Check sheet for the modelled part. Datum: model origin and axes. Units: mm. A direction names the side the tool comes from. Give positions to 0.01 mm unless a question says otherwise; leave off trailing zeros. Write each loop counter-clockwise with the first axis right and the second up, starting at its lowest first coordinate (ties: lowest second). Pieces come first, ordered by that corner, then holes. Notation, with made-up numbers: (-33, 66.25) -> (-8, 66.25) arc R19 cw to (-8, 99.25) -> close; hole circle Ø9 at (-10, -38.5). An arc over 180 degrees is marked (long way). Use a Markdown table: item, result. Add a question column.
1. Release check for a two-part mould opening along X. For faces 1 (the flat face through (2, 12, 15.875)), 2 (the cylindrical face through (21.199, 6.676, 7.826)), 3 (the cylindrical face through (-0.166, 20.637, 7.826)) record: released by +X, released by -X, zero draft, split by the parting line, or undercut.
2. Scan lines: probe 1 along Y at (x, z) = (-0.5, 5.25); probe 2 along X at (y, z) = (8.5, 3.5); probe 3 along X at (y, z) = (3, 14.25). Record each from-to range of solid material in increasing order. Write a range as [from, to].
3. Cross-section at D-D (y = 3). Enter the section's corners in (x, z) (3 decimals).
4. Cross-section at A-A (y = 10.5). Count the separate pieces of the cut face and the enclosed holes in it, then the cut area to 3 significant figures.
5. Cross-section at B-B (x = -5). Enter the section's corners in (y, z) (3 decimals).
6. Gauge pin test, flat ends, axial feed: P1, Ø2, axis at y = 1.5, z = 13.5, coming from the -X side; P2, Ø4, axis at y = -10.5, z = 11.5, coming from the -X side; P3, Ø3, axis at y = -17, z = 8, coming from the +X side. Record the tip position at first contact, or that the pin passes through.
7. Set-up check for faces 4 (the cylindrical face through (10.078, 10.477, 14.265)), 5 (the flat face through (-10, 10, 3.175)), 6 (the cylindrical face through (15.45, 13.31, 6.26)): record each of +Z, -Z, +X, -X, +Y, -Y from which the full face is reachable in a straight line by a thin tool's end or side.
from build123d import *

# Parameters (mm, degrees)
F0_R            = 22.225
F0_R_2          = 2.15265
F1_DEPTH        = 15.875
F4_R            = 3.96875
F5_DEPTH        = 12.7
F6_R            = 3.96875
F7_DEPTH        = 12.7
F9_DEPTH        = 15.875
F9_COPIES_COUNT = 4


# Not quite as in the source:
# - a pattern or mirror of a feature is missing from the dataset's text; its kind, count and spacing are read off the source's solid


with BuildPart() as f1:
    # F0 (on Top) → F1 (new body)
    with BuildSketch(Plane.XY):
        Circle(F0_R)
        with Locations((-11.7865861589, -11.7865861589)):
            Circle(F0_R_2, mode=Mode.SUBTRACT)
        with Locations((11.7865861589, -11.7865861589)):
            Circle(F0_R_2, mode=Mode.SUBTRACT)
        with Locations((-11.7865861589, 11.7865861589)):
            Circle(F0_R_2, mode=Mode.SUBTRACT)
        with BuildLine():
            ThreePointArc((0, 11.1125), (7.8577241059, 7.8577241059), (11.1125, 0))
            ThreePointArc((11.1125, 0), (-7.8577241059, -7.8577241059), (0, 11.1125))
        make_face(mode=Mode.SUBTRACT)
        with Locations((11.7865861589, 11.7865861589)):
            Circle(F0_R_2, mode=Mode.SUBTRACT)
    extrude(amount=F1_DEPTH)

    # F4 (on face) → F5 (cut, through all)
    with BuildSketch(Plane(origin=(0, 0, 0), x_dir=(1, 0, 0), z_dir=(0, 0, -1))):
        with Locations((11.7865861589, -11.7865861589)):
            Circle(F4_R)
        with Locations((-11.7865861589, 11.7865861589)):
            Circle(F4_R)
    extrude(amount=-F5_DEPTH, mode=Mode.SUBTRACT)

    # F6 (on face) → F7 (cut, through all)
    with BuildSketch(Plane.XY.offset(15.875)):
        with Locations((-11.7865861589, 11.7865861589)):
            Circle(F6_R)
        with Locations((11.7865861589, -11.7865861589)):
            Circle(F6_R)
    extrude(amount=-F7_DEPTH, mode=Mode.SUBTRACT)

    # F8 (on face) → F9 (cut, through all)
    with BuildSketch(Plane(origin=(0, 0, 0), x_dir=(1, 0, 0), z_dir=(0, 0, -1))):
        with BuildLine():
            ThreePointArc((-11.229543123, 17.3148424047), (-8.0281867, 15.8788163052), (-6.3255746232, 12.8109235396))
            ThreePointArc((-6.3255746232, 12.8109235396), (0, 14.2875), (6.3255746232, 12.8109235396))
            ThreePointArc((6.3255746232, 12.8109235396), (8.0281867, 15.8788163052), (11.229543123, 17.3148424047))
            ThreePointArc((11.229543123, 17.3148424047), (0, 20.6375), (-11.229543123, 17.3148424047))
        make_face()
    f9 = extrude(amount=-F9_DEPTH, mode=Mode.SUBTRACT)

    # F9_copies: F9 ×4 about axis
    f9_copies_axis = Axis((0, 0, 0), (0, 0, 1))
    for i in range(1, F9_COPIES_COUNT):
        add(f9.rotate(f9_copies_axis, i * 360 / F9_COPIES_COUNT), mode=Mode.SUBTRACT)


solid = f1.part
Worked answers:
| question | item | result |
|---|---|---|
| 1 | face 1 | zero draft |
| 1 | face 2 | split by the parting line |
| 1 | face 3 | undercut |
| 2 | probe 1 | y = [-22.22, -20.63], [-14.28, -11.1], [11.1, 14.28], [20.63, 22.22] |
| 2 | probe 2 | x = [-20.54, -18.81], [-16.27, -14.01], [-9.56, -7.16], [7.16, 9.56], [14.01, 16.27], [18.81, 20.54] |
| 2 | probe 3 | x = [-22.02, -20.42], [-13.97, -10.7], [10.7, 13.97], [20.42, 22.02] |
| 3 | outline | (-22.022, 0) -> (-20.418, 0) -> (-20.418, 15.875) -> (-22.022, 15.875) -> close; (-13.969, 0) -> (-10.7, 0) -> (-10.7, 15.875) -> (-13.969, 15.875) -> close; (10.7, 0) -> (13.969, 0) -> (13.969, 15.875) -> (10.7, 15.875) -> close; (20.418, 0) -> (22.022, 0) -> (22.022, 15.875) -> (20.418, 15.875) -> close |
| 4 | separate pieces | 6 |
| 4 | enclosed holes | 0 |
| 4 | area | 276 mm² |
| 5 | outline | (-21.655, 0) -> (-20.023, 0) -> (-20.023, 15.875) -> (-21.655, 15.875) -> close; (-13.384, 0) -> (-9.924, 0) -> (-9.924, 15.875) -> (-13.384, 15.875) -> close; (9.924, 0) -> (13.384, 0) -> (13.384, 15.875) -> (9.924, 15.875) -> close; (20.023, 0) -> (21.655, 0) -> (21.655, 15.875) -> (20.023, 15.875) -> close |
| 6 | P1 | stops at x = -22.22 |
| 6 | P2 | stops at x = -20.54 |
| 6 | P3 | stops at x = 15.93 |
| 7 | face 4 | +Z, -Z |
| 7 | face 5 | +Z |
| 7 | face 6 | -Z |
